Geometry: final body of the model. Coordinates: model frame, mm. Give positions to 0.01 mm unless a question says otherwise; leave off trailing zeros. Write each loop counter-clockwise with the first axis right and the second up, starting at its lowest first coordinate (ties: lowest second). Pieces come first, ordered by that corner, then holes. Notation, with made-up numbers: (9, 81) - (20, 81) arc R29 cw to (20, 119) - close; hole circle Ø11 at (-38, 24). An arc over 180 degrees is marked (long way). Use CSV: the item, a comma, the result in double quotes. Start each with the question number.
(1) First-contact query: pin 1 Ø2.5 at (x, z) = (6.48, -0.15) entering from -Y; pin 2 Ø2.5 at (x, z) = (6.48, 0.15) entering from -Y; pin 3 Ø4 at (x, z) = (6.48, 0.15) entering from -Y; pin 4 Ø2.5 at (x, z) = (6.5, 0.5) entering from +Y. Flat tips, straight axial feed; report the tip coordinate or a pass-through.
(2) Section C-C on z = -0.5. Count the separate pieces of the cut face and the enclosed holes in it, and give its area (3 significant figures).
(3) Section B-B on x = 19.25. Output: boundary loops of the cut face in (y, z).
(4) Line query: probe 1 along Y at (x, z) = (15, -3); probe 2 along Z at (x, y) = (13.25, 0); probe 3 along Z at (x, y) = (2.75, 6.5). Output: solid intervals per line, ascending. Write a range as [from, to].
(5) Section A-A on x = 10.5. Output: boundary loops of the cut face in (y, z), and give its area (3 significant figures).
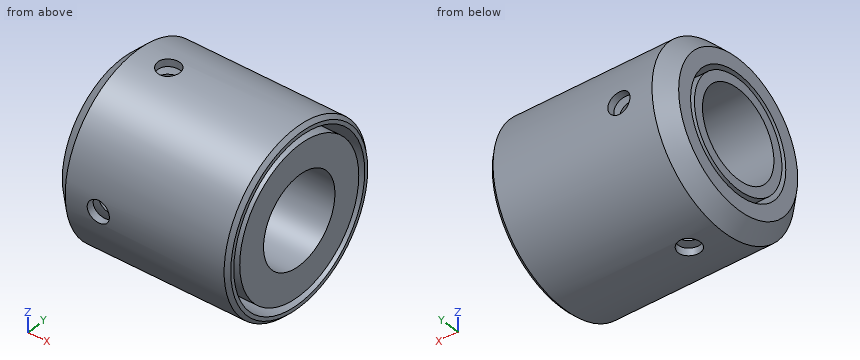
from build123d import *

# Parameters (mm, degrees)
SKETCH017_R           = 12
SKETCH017_R_2         = 6
PAD007_DEPTH          = 12
SKETCH018_R           = 11
SKETCH018_R_2         = 10
POCKET010_DEPTH       = 22
SKETCH019_R           = 8
SKETCH019_R_2         = 7.35
POCKET011_DEPTH       = 13
CHAMFER_SIZE          = 2
CHAMFER001_SIZE       = 0.5
SKETCH020_R           = 1.5
POCKET012_DEPTH       = 5
POLARPATTERN003_COUNT = 4


with BuildPart() as part:
    # Sketch017 → Pad007 (new body, symmetric)
    with BuildSketch(Plane.YZ):
        Circle(SKETCH017_R)
        Circle(SKETCH017_R_2, mode=Mode.SUBTRACT)
    extrude(amount=PAD007_DEPTH, both=True)

    # Sketch018 (on Face4 of Pad007) → Pocket010 (cut)
    with BuildSketch(Plane.YZ.offset(12)):
        Circle(SKETCH018_R)
        Circle(SKETCH018_R_2, mode=Mode.SUBTRACT)
    extrude(amount=-POCKET010_DEPTH, mode=Mode.SUBTRACT)

    # Sketch019 → Pocket011 (cut)
    with BuildSketch(Plane.YZ):
        Circle(SKETCH019_R)
        Circle(SKETCH019_R_2, mode=Mode.SUBTRACT)
    extrude(amount=-POCKET011_DEPTH, mode=Mode.SUBTRACT)

    # Chamfer
    chamfer_edges = [part.edges().sort_by_distance(p)[0] for p in [
        (-12, -12, 0),
    ]]
    chamfer(chamfer_edges, length=CHAMFER_SIZE)

    # Chamfer001
    chamfer001_edges = [part.edges().sort_by_distance(p)[0] for p in [
        (12, -12, 0),
    ]]
    chamfer(chamfer001_edges, length=CHAMFER001_SIZE)

    # Sketch020 → Pocket012 (cut)
    with BuildSketch(Plane.XY.offset(-12)):
        with Locations((-5.524041, 0.1487)):
            Circle(SKETCH020_R)
    pocket012 = extrude(amount=POCKET012_DEPTH, mode=Mode.SUBTRACT)

    # PolarPattern003: Pocket012 ×4 about axis
    polarpattern003_axis = Axis((0, 0, 0), (1, 0, 0))
    for i in range(1, POLARPATTERN003_COUNT):
        add(pocket012.rotate(polarpattern003_axis, i * 360 / POLARPATTERN003_COUNT), mode=Mode.SUBTRACT)


with BuildPart() as part_1:
    # Body003 placement: moved
    add(part.part.moved(Location((12, 0, 0))))


solid = part_1.part
Check values:
1,pin 1,"stops at y = -7"
1,pin 2,"stops at y = -11.95"
1,pin 3,"stops at y = -12"
1,pin 4,"stops at y = 11.94"
2,separate pieces,"6"
2,enclosed holes,"0"
2,area,"206 mm²"
3,outline,"circle Ø24 at (0, 0); circle Ø20 at (0, 0); hole circle Ø22 at (0, 0); hole circle Ø12 at (0, 0)"
4,probe 1,"y = [-11.62, -10.58], [-9.54, -5.2], [5.2, 9.54], [10.58, 11.62]"
4,probe 2,"z = [-12, -11], [-10, -6], [6, 10], [11, 12]"
4,probe 3,"z = [-10.09, -8.87], [-7.6, -4.66], [-3.43, 3.43], [4.66, 7.6], [8.87, 10.09]"
5,outline,"circle Ø24 at (0, 0); circle Ø20 at (0, 0); circle Ø14.7 at (0, 0); hole circle Ø22 at (0, 0); hole circle Ø16 at (0, 0); hole circle Ø12 at (0, 0)"
5,area,"242 mm²"
